```python
from build123d import *

# Parameters (mm, degrees)
F1_ANGLE      = 180
F2_R          = 3.9973769872
F2_R_2        = 3.614591246
F3_DEPTH      = 7.2390632276
F3_DEPTH_BACK = 25.4


with BuildPart() as f1:
    # F0 (on Top) → F1 (revolve)
    with BuildSketch(Plane.XY):
        with BuildLine():
            add(Edge.make_bspline(
                [(0, 0), (23.9424614, 3.6743346017), (70.7544254358, 10.8583432184), (114.3867719938, 3.5637158267), (135.7029080391, 0)],
                knots=[0, 0, 0, 0, 0.5114602064, 1, 1, 1, 1], degree=3))
            Line((0, 0), (135.7029080391, 0))
        make_face()
    revolve(axis=Axis((67.8514540195, 0, 0), (1, 0, 0)), revolution_arc=F1_ANGLE)

    # F2 (on Front) → F3 (cut, two sides)
    with BuildSketch(Plane.XZ) as f3_sk:
        with Locations((54.1759431362, 0)):
            Circle(F2_R)
        with Locations((90.7356441021, 0)):
            Circle(F2_R_2)
    extrude(amount=F3_DEPTH, mode=Mode.SUBTRACT)
    extrude(f3_sk.sketch, amount=-F3_DEPTH_BACK, mode=Mode.SUBTRACT)


solid = f1.part
```
Here's how the part is built. I have some questions about the finished solid (model axes, mm). Give positions to 0.01 mm unless a question says otherwise; leave off trailing zeros. Answer as a JSON object with one key per item and string values. Group by question number.
Item 1: If we section it at A-A on z = 2.5: Give the number of separate pieces and of enclosed holes in the cut face, and give its area (3 significant figures).
Item 2: For P1, Ø1, axis at x = 67.5, z = 3.5, coming from the +Y side; P2, Ø1, axis at x = 90.5, y = -1.5, coming from the -Z side, each with a flat end and sliding along its axis, tell me the tip position at first contact or that it passes through.
Item 3: Please list where these lines run through material, in increasing order: probe 1 along Z at (x, y) = (54, 1.75); probe 2 along Y at (x, z) = (130, 0.5); probe 3 along Y at (x, z) = (68, 5).
Result set:
{
 "1": {"separate pieces": "3", "enclosed holes": "0", "area": "865 mm²"},
 "2": {"P1": "y = 6.57", "P2": "z = 3.54"},
 "3": {"probe 1": "3.99 to 6.47", "probe 2": "-0.81 to 0.81", "probe 3": "-5.22 to 5.22"}
}
